Autodesk Inventor part; units mm, degrees
ref_plane "YZ Plane" through (0, 0, 0) normal (1, 0, 0) x (0, 1, 0)
ref_plane "XZ Plane" through (0, 0, 0) normal (0, 1, 0) x (-1, 0, 0)
ref_plane "XY Plane" through (0, 0, 0) normal (0, 0, 1) x (1, 0, 0)
sketch "Sketch1" plane through (0, 0, 0) normal (0, 0, 1) x (1, 0, 0)
  line L0 (0, 0) -> (10, 0)
  line L1 (10, 0) -> (10, 3.175)
  line L2 (10, 3.175) -> (24.605, 3.175)
  line L3 (24.605, 3.175) -> (24.605, 0)
  line L4 (24.605, 0) -> (34.605, 0)
  line L5 (0, 2) -> (8, 2)
  line L6 (8, 2) -> (8, 5.175)
  line L7 (8, 5.175) -> (26.605, 5.175)
  line L8 (26.605, 5.175) -> (26.605, 2)
  line L9 (26.605, 2) -> (34.605, 2)
  line L10 (0, 2) -> (0, 0)
  line L11 (34.605, 0) -> (34.605, 2)
  dimension "d0" = 10
  dimension "d1" = 3.175
  dimension "d2" = 14.605
  dimension "d3" = 10
  dimension "d4" = 2
extrude "Extrusion1" add sketch "Sketch1" along normal blind 43.18
sketch "Sketch2" plane through (10, 3.175, 0) normal (0, -1, 0) x (1, 0, 0)
  line L0 (0, 0) -> (14.605, 0)
  line L1 (14.605, 0) -> (14.605, 43.18)
  line L2 (0, 43.18) -> (14.605, 43.18)
  line L3 (0, 0) -> (0, 43.18)
  line L4 (14.605, 0) -> (14.605, 43.18)
  line L5 (14.605, 0) -> (14.605, 6.985)
  line L6 (14.605, 6.985) -> (12.065, 6.985)
  circle A0 centre (12.065, 6.985) radius 1.3891
  line L7 (0, 0) -> (14.605, 0)
  line L8 (0, 0) -> (0, 6.985)
  line L9 (0, 0) -> (0, 43.18)
  line L10 (0, 6.985) -> (2.54, 6.985)
  circle A1 centre (2.54, 6.985) radius 1.3891
  line L11 (14.605, 43.18) -> (14.605, 36.195)
  line L12 (14.605, 36.195) -> (12.065, 36.195)
  circle A2 centre (12.065, 36.195) radius 1.3891
  line L13 (-10, 43.18) -> (0, 43.18)
  line L14 (0, 43.18) -> (0, 36.195)
  line L15 (0, 36.195) -> (2.54, 36.195)
  circle A3 centre (2.54, 36.195) radius 1.3891
  point P0 (-10, 0)
  dimension "d7" = 6.985
  dimension "d8" = 2.54
  dimension "d9" = 2.7781
  dimension "d10" = 6.985
  dimension "d11" = 2.54
  dimension "d12" = 2.7781
  dimension "d13" = 6.985
  dimension "d14" = 2.54
  dimension "d15" = 2.7781
  dimension "d16" = 6.985
  dimension "d17" = 2.54
  dimension "d18" = 2.7781
extrude "Extrusion2" cut sketch "Sketch2" against normal blind 43.18 contours A0 | A2 | A3 | A1
fillet "Fillet1" radius 4 4 edges at (34.605, 1, 43.18) (34.605, 1, 0) (0, 1, 0) (0, 1, 43.18)
sketch "Sketch4" plane through (26.605, 2, 43.18) normal (0, 1, 0) x (1, 0, 0)
  arc A0 (-26.605, 4) -> (-22.605, 0) centre (-22.605, 4) ccw
  arc A1 (-22.605, 43.18) -> (-26.605, 39.18) centre (-22.605, 39.18) ccw
  arc A2 (8, 39.18) -> (4, 43.18) centre (4, 39.18) ccw
  arc A3 (4, 0) -> (8, 4) centre (4, 4) ccw
  circle A4 centre (4, 4) radius 2.1
  circle A5 centre (4, 39.18) radius 2.1
  circle A6 centre (-22.605, 39.18) radius 2.1
  circle A7 centre (-22.605, 4) radius 2.1
  point P0 (-26.605, 43.18)
  dimension "d22" = 4.2
  dimension "d23" = 4.2
  dimension "d24" = 4.2
  dimension "d25" = 4.2
extrude "Extrusion3" cut sketch "Sketch4" against normal blind 43.18
properties part number "buckconverter-holder"
Could you check a few things on this model? Use its own coordinates, in mm. A direction names the side the tool comes from. Coordinates: 2 decimals unless noted, no trailing zeros. Order: outer loops, then holes, each group sorted by start corner. A loop starts at its lowest first (then second) coordinate and runs counter-clockwise, first axis right, second up. Notation, with made-up numbers: M 45,-35.75 L 104,-35.75 A26 cw 104,1.25 Z; hole C 19.5,19.25 d8. An arc over 180 degrees is marked long. Use a Markdown table: item, result. Add a question column.
Q1. I want a section at B-B on z = 13.5. List the corners of the cut face in (x, y) for me (3 decimals).
Q2. I want a section at A-A on y = 0.9. List the corners of the cut face in (x, z) for me (3 decimals).
Q3. I'm going to push flat-ended pins straight in: pin 1 (5.5 mm diameter, centred on x = 30.605, z = 4, fed in from +Y); pin 2 (2.5 mm diameter, centred on y = 2.5, z = 24.5, fed in from -X); pin 3 (1 mm diameter, centred on y = 4, z = 11.5, fed in from +X) (3 decimals); pin 4 (6 mm diameter, centred on x = 20, z = 32.5, fed in from -Y) (3 decimals). Where does each tip first touch, or does it pass through?
Q4. We'd pull the mould along Z, two halves only. Please class faces 4 (the flat face through (10, 2, 21)), 5 (the cylindrical face through (21.76, 4.16, 34.84)), 6 (the cylindrical face through (1.141, 0.986, 1.203)): pulls with the +Z half, pulls with the -Z half, needs draft (parallel to the pull), parting line crosses it, or undercut.
Q5. I want a section at C-C on y = 3.8. List the corners of the cut face in (x, z) for me (3 decimals).
Q6. If I drill on L1, parallel to X at y = 1.35, z = 39.18 (3 decimals); L2, parallel to X at y = 0.25, z = 17 (3 decimals); L3, parallel to X at y = 2.4, z = 2.5 (3 decimals), over which ranges is the centre line in solid material (lowest first)?
Q7. Which directions (+Z, -Z, +X, -X, +Y, -Y) give clear straight access to the entire face, cutting with the end or side of a thin tool? Please do faces 1 (the flat face through (17, 3.175, 21)), 2 (the flat face through (8, 4, 21)), 3 (the cylindrical face through (3.7, 1, 37.1)).
Checked values:
| question | item | result |
|---|---|---|
| 1 | outline | M 0,0 L 10,0 L 10,3.175 L 24.605,3.175 L 24.605,0 L 34.605,0 L 34.605,2 L 26.605,2 L 26.605,5.175 L 8,5.175 L 8,2 L 0,2 Z |
| 2 | outline | M 0,4 A4 ccw 4,0 L 10,0 L 10,43.18 L 4,43.18 A4 ccw 0,39.18 Z; M 24.605,0 L 30.605,0 A4 ccw 34.605,4 L 34.605,39.18 A4 ccw 30.605,43.18 L 24.605,43.18 Z; hole C 4,4 d4.2; hole C 4,39.18 d4.2; hole C 30.605,4 d4.2; hole C 30.605,39.18 d4.2 |
| 3 | pin 1 | y = 2 |
| 3 | pin 2 | x = 0 |
| 3 | pin 3 | x = 26.605 |
| 3 | pin 4 | y = 3.175 |
| 4 | face 4 | needs draft |
| 4 | face 5 | undercut |
| 4 | face 6 | pulls with the -Z half |
| 5 | outline | M 8,0 L 26.605,0 L 26.605,43.18 L 8,43.18 Z; hole C 12.54,6.985 d2.778; hole C 12.54,36.195 d2.778; hole C 22.065,6.985 d2.778; hole C 22.065,36.195 d2.778 |
| 6 | L1 | 0 to 1.9, 6.1 to 10, 24.605 to 28.505, 32.705 to 34.605 |
| 6 | L2 | 0 to 10, 24.605 to 34.605 |
| 6 | L3 | 8 to 10, 24.605 to 26.605 |
| 7 | face 1 | +Z, -Z, -Y |
| 7 | face 2 | +Z, -Z, -X, +Y |
| 7 | face 3 | +Y, -Y |
